Check sheet for the modelled part. Datum: model origin and axes. Units: mm. Face numbers are marked on the shaded views. A direction names the side the tool comes from. Give positions to 0.01 mm unless a question says otherwise; leave off trailing zeros. Write each loop counter-clockwise with the first axis right and the second up, starting at its lowest first coordinate (ties: lowest second). Pieces come first, ordered by that corner, then holes. Notation, with made-up numbers: M 62.5,66.25 L 68.5,66.25 A5 ccw 68.5,70.25 Z; hole C 4,61.5 d2. An arc over 180 degrees is marked long. Write item = value, one per line. Start each with the question number.
1) Sectioned sample at B-B, the plane x = -1. Count the separate pieces of the cut face and the enclosed holes in it, then the cut area to 3 significant figures.
2) Scan lines: L1, parallel to X at y = -21, z = 33.5; L2, parallel to Y at x = -19.5, z = 21; L3, parallel to X at y = -7, z = 24.5. Record each from-to range of solid material in increasing order.
3) Set-up check for the marked faces 4, 5, 6 and 7: record each of +Z, -Z, +X, -X, +Y, -Y from which the full face is reachable in a straight line by a thin tool's end or side.
4) Gauge pin test, flat ends, axial feed: pin 1 (3 mm diameter, centred on y = -15.21, z = 6.29, fed in from +X); pin 2 (12 mm diameter, centred on x = -21.5, z = 35, fed in from -Y); pin 3 (5 mm diameter, centred on y = 8.5, z = 24, fed in from +X); pin 4 (2 mm diameter, centred on y = 38, z = 32.5, fed in from +X). Record the tip position at first contact, or that the pin passes through.
5) Sectioned sample at C-C, the plane z = 12.5. Record the cut outline in (x, y).
6) Sectioned sample at A-A, the plane y = 18.5. Record the cut outline in (x, z), then the cut area to 3 significant figures.
7) Draft check along Y on the marked faces 1, 2 and 3. Enter one of: pulls with the +Y half, pulls with the -Y half, needs draft (parallel to the pull), parting line crosses it, or undercut.
8) Sectioned sample at D-D, the plane y = 35.5. Record the cut outline in (x, z), then the cut area to 3 significant figures.
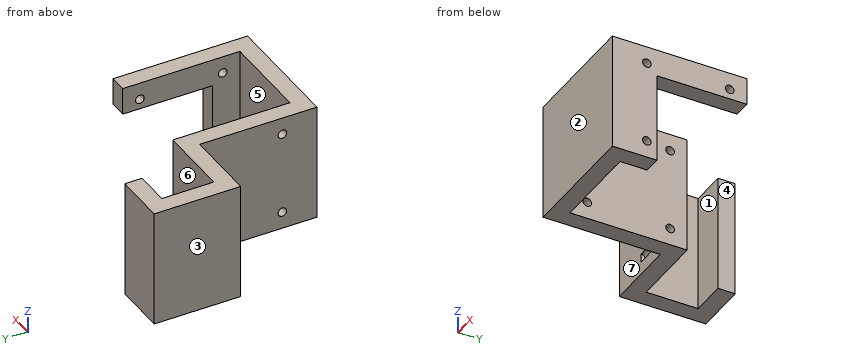
from build123d import *

# Parameters (mm, degrees)
BOSS_EXTRUDE1_DEPTH     = 43
SKETCH2_W               = 33
SKETCH2_H               = 6.35
SKETCH2_H_2             = 10
SKETCH2_R               = 1.5
SKETCH2_W_2             = 10
BOSS_EXTRUDE2_DEPTH     = 6.35
CUT_EXTRUDE1_DEPTH      = 79.339645136
CUT_EXTRUDE1_DEPTH_BACK = 12.7
SKETCH3_R               = 1.5875


with BuildPart() as part:
    # Sketch1 → Boss-Extrude1 (new body)
    with BuildSketch(Plane.XY):
        Polygon((-6.35, -27.85), (-6.35, 15.15), (-33.4, 15.15), (-33.4, 46.9), (-14, 46.9), (-14, 40.55), (-27.05, 40.55), (-27.05, 21.5), (0, 21.5), (0, -21.5), (33, -21.5), (33, -27.85), align=None)
    extrude(amount=-BOSS_EXTRUDE1_DEPTH)

    # Sketch2 → Boss-Extrude2 (add)
    # profile 1 of 4: a face of its own
    with BuildSketch(Plane(origin=(33, 0, 0), x_dir=(0, 0, -1), z_dir=(1, 0, 0))):
        with Locations((16.5, -24.675)):
            Rectangle(SKETCH2_W, SKETCH2_H)
    # profile 2 of 4: a face of its own
    with BuildSketch(Plane(origin=(33, 0, 0), x_dir=(0, 0, -1), z_dir=(1, 0, 0))):
        with Locations((16.5, -16.5)):
            Rectangle(SKETCH2_W, SKETCH2_H_2)
        with Locations((6.294174233, -15.205825767)):
            Circle(SKETCH2_R, mode=Mode.SUBTRACT)
    # profile 3 of 4: a face of its own
    with BuildSketch(Plane(origin=(33, 0, 0), x_dir=(0, 0, -1), z_dir=(1, 0, 0))):
        with Locations((38, -24.675)):
            Rectangle(SKETCH2_W_2, SKETCH2_H)
    # profile 4 of 4: a face of its own
    with BuildSketch(Plane(origin=(33, 0, 0), x_dir=(0, 0, -1), z_dir=(1, 0, 0))):
        Polygon((33, -11.5), (33, -21.5), (43, -21.5), (43, 21.5), (33, 21.5), align=None)
        with Locations((36.705825767, -15.205825767)):
            Circle(SKETCH2_R, mode=Mode.SUBTRACT)
        with Locations((36.705825767, 15.205825767)):
            Circle(SKETCH2_R, mode=Mode.SUBTRACT)
    extrude(amount=BOSS_EXTRUDE2_DEPTH)

    # Sketch3 → Cut-Extrude1 (cut, two sides: drawn at the far end of the back side and taken through both)
    with BuildSketch(Plane(origin=(-6.35, 0, 0), x_dir=(0, 0, -1), z_dir=(1, 0, 0)).offset(-CUT_EXTRUDE1_DEPTH_BACK)):
        with Locations(Location((6.294174233, -15.205825767, 0), (0, 0, 270))):
            Circle(SKETCH3_R)
        with Locations(Location((6.294174233, 15.205825767, 0), (0, 0, 270))):
            Circle(SKETCH3_R)
        with Locations(Location((36.705825767, 15.205825767, 0), (0, 0, 270))):
            Circle(SKETCH3_R)
        with Locations(Location((36.705825767, -15.205825767, 0), (0, 0, 270))):
            Circle(SKETCH3_R)
    extrude(amount=CUT_EXTRUDE1_DEPTH + CUT_EXTRUDE1_DEPTH_BACK, mode=Mode.SUBTRACT)


with BuildPart() as body_2:
    # Mirror1: mirrored copy
    add(part.part.mirror(Plane.XY))


solid = body_2.part
Data:
q1.separate_pieces = 1
q1.enclosed_holes = 4
q1.area = 2,090 mm2
q2.L1 = -6.35 to 0, 33 to 39.35
q2.L2 = 15.15 to 21.5, 40.55 to 46.9
q2.L3 = -6.35 to 0
q3.face_4 = +Z, -Z, +X, +Y
q3.face_5 = +Z, -Z, +Y
q3.face_6 = +Z, -Z, +X
q3.face_7 = +Z, -Z, -X, -Y
q4.pin_1 = through
q4.pin_2 = 15.15
q4.pin_3 = 0
q4.pin_4 = -27.05
q5.outline = M -33.4,15.15 L -6.35,15.15 L -6.35,-27.85 L 39.35,-27.85 L 39.35,-11.5 L 33,-11.5 L 33,-21.5 L 0,-21.5 L 0,21.5 L -27.05,21.5 L -27.05,40.55 L -14,40.55 L -14,46.9 L -33.4,46.9 Z
q6.outline = M -33.4,0 L 0,0 L 0,43 L -33.4,43 Z; M 33,33 L 39.35,33 L 39.35,43 L 33,43 Z
q6.area = 1,500 mm2
q7.face_1 = undercut
q7.face_2 = pulls with the -Y half
q7.face_3 = needs draft
q8.outline = M -33.4,0 L -27.05,0 L -27.05,43 L -33.4,43 Z
q8.area = 273 mm2
